from build123d import *

# Parameters (mm, degrees)
F0_W     = 9.4753347638
F0_H     = 30
F0_R     = 17.5
F1_DEPTH = 15
F2_R     = 2
F3_R     = 2


# Not quite as in the source:
# - a feature names something its author has since deleted; it is built from what else it names


with BuildPart() as f1:
    # F0 (on Top) → F1 (new body)
    with BuildSketch(Plane.XY):
        with Locations((-149.2113988997, 5.7397255301)):
            Rectangle(F0_W, F0_H)
        Polygon((1.0509337184, 20.7397255301), (1.0509337184, 45.7397255301), (-153.9490662816, 45.7397255301), (-153.9490662816, 20.7397255301), (-144.4737315178, 20.7397255301), (-135.1745359898, 20.7397255301), (-134.4737315178, 20.7397255301), (-127.1745359898, 20.7397255301), (-117.1745359898, 20.7397255301), (-103.1745359898, 20.7397255301), align=None)
        with BuildLine():
            ThreePointArc((1.0509337184, 20.7397255301), (68.742675795, 33.2397255301), (1.0509337184, 45.7397255301))
            Line((1.0509337184, 45.7397255301), (1.0509337184, 20.7397255301))
        make_face()
        with Locations((33.742675795, 33.2397255301)):
            Circle(F0_R, mode=Mode.SUBTRACT)
        Polygon((-134.4737315178, 20.7397255301), (-135.1745359898, 20.7397255301), (-135.1745359898, 5.7397255301), (-134.4737315178, 5.7397255301), (-127.1745359898, 5.7397255301), (-127.1745359898, 20.7397255301), align=None)
        Polygon((-110.1745359898, 5.7397255301), (-103.1745359898, 20.7397255301), (-117.1745359898, 20.7397255301), align=None)
    extrude(amount=F1_DEPTH)

    # F2
    f2_edges = [f1.edges().sort_by_distance(p)[0] for p in [
        (68.742676, 33.239726, 0),
        (16.242676, 33.239726, 0),
        (-51.061801, 20.739726, 0),
        (-106.674536, 13.239726, 0),
        (-127.174536, 13.239726, 0),
        (-122.174536, 20.739726, 0),
        (-113.674536, 13.239726, 0),
        (-135.174536, 13.239726, 0),
        (-131.174536, 5.739726, 0),
        (-139.824134, 20.739726, 0),
        (-144.473732, 5.739726, 0),
        (-149.211399, -9.260274, 0),
        (-153.949066, 18.239726, 0),
    ]]
    fillet(f2_edges, radius=F2_R)

    # F3
    f3_edges = [f1.edges().sort_by_distance(p)[0] for p in [
        (-149.211399, -9.260274, 15),
        (-144.473732, 5.739726, 15),
        (-139.824134, 20.739726, 15),
        (-135.174536, 13.239726, 15),
        (-131.174536, 5.739726, 15),
        (-127.174536, 13.239726, 15),
        (-122.174536, 20.739726, 15),
        (-113.674536, 13.239726, 15),
        (-106.674536, 13.239726, 15),
        (-51.061801, 20.739726, 15),
        (68.742676, 33.239726, 15),
        (-76.449066, 45.739726, 15),
        (-153.949066, 18.239726, 15),
        (16.242676, 33.239726, 15),
    ]]
    fillet(f3_edges, radius=F3_R)


solid = f1.part
The model under review builds one solid part; all positions refer to its coordinate system, in mm. A direction names the side the tool comes from. Round coordinates to 2 decimals unless told otherwise and drop trailing zeros. Order: outer loops, then holes, each group sorted by start corner. A loop starts at its lowest first (then second) coordinate and runs counter-clockwise, first axis right, second up. Notation, with made-up numbers: (85, 24) -> (108, 24) arc R9 ccw to (108, 29) -> close; hole circle Ø11 at (13.25, 13.25). An arc over 180 degrees is marked (long way). Use CSV: the item, a comma, the result in double quotes. Start each with the question number.
(1) Consider section A-A on x = -47. Write out the cut boundary in (y, z), and give its area (3 significant figures).
(2) Tool access review of faces 1 (the face through (-106.87, 14.17, 14.4)), 2 (the face through (-74, 45.74, 6)), 3 (the face through (-140, 20.74, 7)): name each direction out of +Z, -Z, +X, -X, +Y, -Y from which nothing blocks a thin tool from reaching the whole face with its end or side.
(3) Insertion check: pin 1 (4 mm diameter, centred on y = 48.5, z = 3, fed in from -X); pin 2 (3 mm diameter, centred on x = -109.5, y = 8, fed in from +Z); pin 3 (5.5 mm diameter, centred on y = -0.5, z = 7.5, fed in from +X). Each pin has a flat end and moves straight along its axis. Give the tip position at first contact, or say it passes through.
(4) Mouldability with a two-part tool opening along X and no side actions: class faces 4 (the face through (41.818, 17.714, 7.423)), 5 (the face through (-35, 32, 0)), 6 (the face through (-153.949, 19, 7)) as pulls with the +X half, pulls with the -X half, needs draft (parallel to the pull), parting line crosses it, or undercut.
(5) Wall thickness on probe 1 along X at (y, z) = (5, 9); probe 2 along Y at (x, z) = (-53.5, 10); probe 3 along Y at (x, z) = (29.5, 4.75): over which ranges is each line inside the solid? List them lowest first. Write a range as from..to.
Responses:
1,outline,"(20.74, 2) arc R2 ccw to (22.74, 0) -> (45.74, 0) -> (45.74, 13) arc R2 ccw to (43.74, 15) -> (22.74, 15) arc R2 ccw to (20.74, 13) -> close"
1,area,"372 mm²"
2,face 1,"+Z, -Y"
2,face 2,"+Z, -Z, -X, +Y"
2,face 3,"+Z, -Z, -Y"
3,pin 1,"x = 1.35"
3,pin 2,"z = 14.94"
3,pin 3,"x = 50.01"
4,face 4,"undercut"
4,face 5,"needs draft"
4,face 6,"pulls with the -X half"
5,probe 1,"-153.95..-144.47, 13.07..54.42"
5,probe 2,"20.74..45.74"
5,probe 3,"-1.5..16.26, 50.22..67.98"
